from build123d import *

# Parameters (mm, degrees)
PAD_DEPTH = 580


with BuildPart() as part:
    # Sketch → Pad (new body)
    with BuildSketch(Plane.XZ):
        Polygon((-7.5, 0), (7.5, 0), (7.5, 2.7), (5, 5.2), (5, 7.2), (7.5, 9.7), (7.5, 12.5), (5, 15), (-5, 15), (-7.5, 12.5), (-7.5, 9.7), (-5, 7.2), (-5, 5.2), (-7.5, 2.7), align=None)
    extrude(amount=PAD_DEPTH)


solid = part.part
Geometry: final body of the model. Coordinates: model frame, mm. Coordinates: 2 decimals unless noted, no trailing zeros. Loops run counter-clockwise (first coordinate to the right, second up) from the corner with the lowest first, then second, coordinate; pieces in that order, holes last. Notation, with made-up numbers: M -20,-32.75 L 4,-32.75 A22 ccw 4,-15.75 Z; hole C 16.25,-8 d1. An arc over 180 degrees is marked long. One line per item, written item: value. Start each with the question number.
1) Pin query (flat end, axial travel): P1, Ø0.6, axis at y = -297.5, z = 6, coming from the +X side; P2, Ø3, axis at x = -2, y = -374, coming from the -Z side; P3, Ø1, axis at y = -60.5, z = 7.5, coming from the +X side; P4, Ø1, axis at y = -420.5, z = 6, coming from the -X side. Return the tip coordinate at first contact, or that it passes through.
2) Cut plane A-A (y = -407.5). Return loops of the section in (x, z).
3) Material intervals for L1, parallel to X at y = -507, z = 5.5; L2, parallel to X at y = -292, z = 7.25; L3, parallel to Z at x = 5.5, y = -352.5, sorted ascending. Write a range as from..to.
Evaluation:
1. P1: x = 5
1. P2: z = 0
1. P3: x = 5.8
1. P4: x = -5
2. outline: M -7.5,0 L 7.5,0 L 7.5,2.7 L 5,5.2 L 5,7.2 L 7.5,9.7 L 7.5,12.5 L 5,15 L -5,15 L -7.5,12.5 L -7.5,9.7 L -5,7.2 L -5,5.2 L -7.5,2.7 Z
3. L1: -5..5
3. L2: -5.05..5.05
3. L3: 0..4.7, 7.7..14.5
